Autodesk Inventor part; units mm, degrees
ref_plane "YZ Plane" through (0, 0, 0) normal (1, 0, 0) x (0, 1, 0)
ref_plane "XZ Plane" through (0, 0, 0) normal (0, 1, 0) x (-1, 0, 0)
ref_plane "XY Plane" through (0, 0, 0) normal (0, 0, 1) x (1, 0, 0)
sketch "スケッチ1" plane through (0, 0, 0) normal (0, 1, 0) x (-1, 0, 0)
  line L0 (8.1505, 14.0302) -> (-11.8495, 14.0302)
  line L1 (-11.8495, 14.0302) -> (-11.8495, -13.0164)
  line L2 (-11.8495, -13.0164) -> (8.1505, -13.0164)
  line L3 (8.1505, -13.0164) -> (8.1505, 14.0302)
  point P0 (0, 0)
  dimension "d0" = 20
extrude "押し出し1" add sketch "スケッチ1" along normal blind 20
sketch "スケッチ2" plane through (-8.1505, 0, 14.0302) normal (0, 0, 1) x (1, 0, 0)
  point P0 (8.1505, 0)
sketch "スケッチ3" plane through (11.8495, 0, -13.0164) normal (0, 0, -1) x (-1, 0, 0)
  circle A0 centre (10, 10) radius 3
  line L0 (0, 20) -> (20, 20)
  line L1 (20, 0) -> (20, 20)
  point P0 (11.8495, 0)
  dimension "d3" = 6
  dimension "d4" = 10
  dimension "d5" = 10
hole "穴1" at (1.8495, 10, -13.0164) direction (0, 0, 1) diameter 6 depth 10
sketch "スケッチ4" plane through (0, 20, 0) normal (0, 1, 0) x (1, 0, 0)
  circle A0 centre (1.8456, -14.0152) radius 10
  point P0 (0, 0)
  dimension "d13" = 20
hole "穴2" at (1.8456, 20, 14.0152) direction (0, -1, 0) diameter 20 depth 20
sketch "スケッチ5" plane through (0, 20, 0) normal (0, 1, 0) x (1, 0, 0)
  circle A0 centre (1.6726, -19.0329) radius 15
  point P0 (0, 0)
  dimension "d21" = 30
hole "穴3" at (1.6726, 20, 19.0329) direction (0, -1, 0) diameter 30 depth 30
equation "\"BendRadius\" = Thickness"
equation "\"BendReliefWidth\" = Thickness"
equation "\"BendReliefDepth\" = 0.5 * Thickness"
equation "\"CornerReliefSize\" = 4 * Thickness"
equation "\"MinimumRemnant\" = 2 * Thickness"
equation "\"TransitionRadius\" = BendRadius"
equation "\"JacobiRadiusSize\" = BendRadius"
equation "\"GapSize\" = Thickness"
The model under review builds one solid part; all positions refer to its coordinate system, in mm. A direction names the side the tool comes from. Give positions to 0.01 mm unless a question says otherwise; leave off trailing zeros. Write each loop counter-clockwise with the first axis right and the second up, starting at its lowest first coordinate (ties: lowest second). Pieces come first, ordered by that corner, then holes. Notation, with made-up numbers: M 29.5,51.25 L 87.5,51.25 A13 ccw 87.5,65.25 Z; hole C 46,82 d4. An arc over 180 degrees is marked long. One line per question, with ' | ' between items. Start each with the question number.
Item 1: We need section A-A on y = 10. Write out the cut boundary in (x, z), plus the area to 3 significant figures.
Item 2: Draft analysis for pull direction X (two halves, no side actions). For faces 1 (the cylindrical face through (7.825, 9.86, 5.353)), 2 (the flat face through (-8.15, 10, -3)), 3 (the flat face through (11.85, 10, -2)), state which applies: released by +X, released by -X, zero draft, split by the parting line, or undercut.
Item 3: We need section D-D on y = 12. Write out the cut boundary in (x, z), plus the area to 3 significant figures.
Item 4: We need section B-B on z = -5. Write out the cut boundary in (x, y).
Item 5: For faces 4 (the flat face through (2, 10, -3.016)), 5 (the cylindrical face through (-3.91, 9.86, 5.11)), 6 (the flat face through (2, 20, -5)), list the 3-axis set-ups (+Z, -Z, +X, -X, +Y, -Y) from which the entire face can be reached by the end or side of a thin tool; tool diameter is ignored.
Item 6: For pin 1 (5 mm diameter, centred on x = -4.5, y = 2.5, fed in from +Z), flat-tipped, find the tip position at first contact; note if it passes through.
Item 7: Wall thickness on line 1 (X direction, y = 10, z = -8.25); line 2 (Z direction, x = 1, y = 11.75); line 3 (Y direction, x = 2.5, z = -8): over which ranges is each line inside the solid? List them lowest first. Write a range as from..to.
Item 8: We need section C-C on x = 3.75. Write out the cut boundary in (y, z).
Results found:
1) outline: M -8.15,-13.02 L -1.15,-13.02 L -1.15,-3.02 L 4.85,-3.02 L 4.85,-13.02 L 11.85,-13.02 L 11.85,8.01 A15 cw 3.3,4.12 A10 cw 1.08,4.04 A15 cw -8.15,7.7 Z | area: 305 mm2
2) face 1: undercut | face 2: released by -X | face 3: released by +X
3) outline: M -8.15,-13.02 L -0.39,-13.02 L -0.39,-3.02 L 4.09,-3.02 L 4.09,-13.02 L 11.85,-13.02 L 11.85,8.01 A15 cw 3.3,4.12 A10 cw 1.08,4.04 A15 cw -8.15,7.7 Z | area: 320 mm2
4) outline: M -8.15,0 L 11.85,0 L 11.85,20 L -8.15,20 Z; hole C 1.85,10 d6
5) face 4: -Z | face 5: +Z, +Y, -Y | face 6: +Z, -Z, +X, -X, +Y
6) pin 1: stops at z = 6.79
7) line 1: x = -8.15..-1.15, 4.85..11.85 | line 2: z = -3.02..4.05 | line 3: y = 0..7.07, 12.93..20
8) outline: M 0,-13.02 L 7.68,-13.02 L 7.68,-3.02 L 12.32,-3.02 L 12.32,-13.02 L 20,-13.02 L 20,4.18 L 0,4.18 Z
